Verification items for this drawing (mm, ordinates from the low corner). A direction names the side the tool comes from. Round coordinates to 2 decimals unless told otherwise and drop trailing zeros. Loops run counter-clockwise (first coordinate to the right, second up) from the corner with the lowest first, then second, coordinate; pieces in that order, holes last. Notation, with made-up numbers: M 42.25,37.5 L 93.25,37.5 A15 ccw 93.25,47.5 Z; hole C 54.5,41.25 d6. An arc over 180 degrees is marked long. One line per item, written item: value.
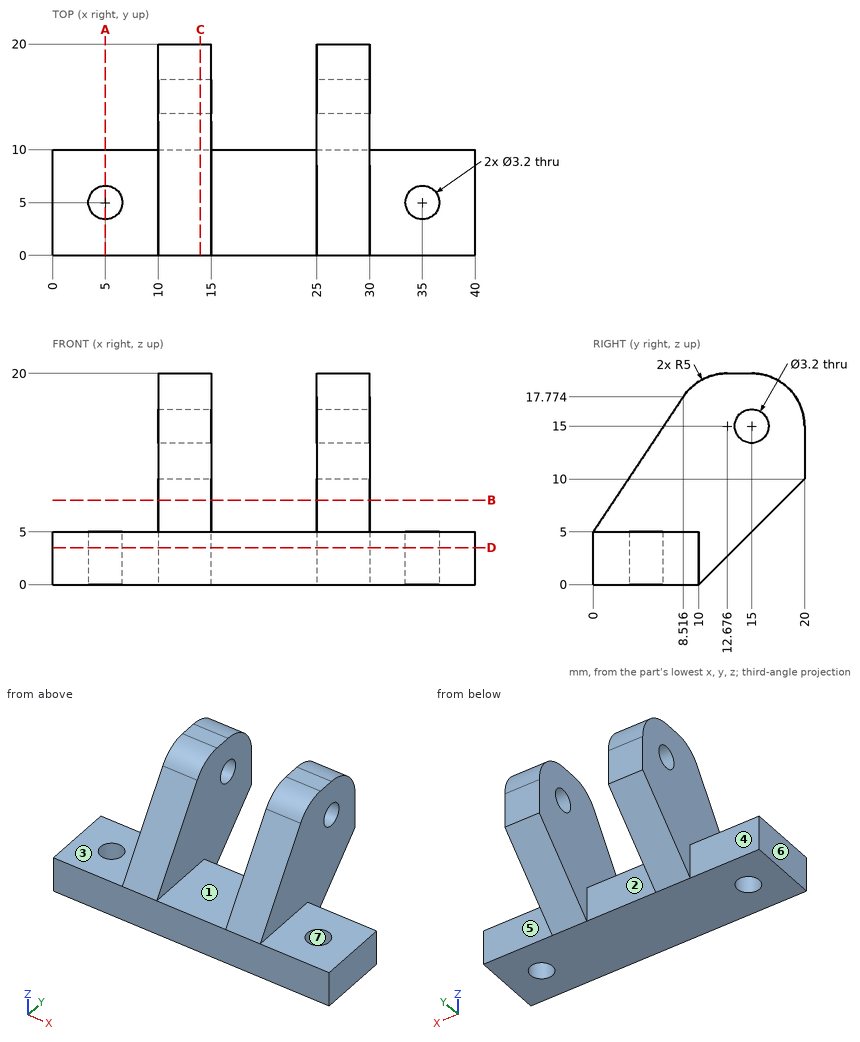
(1) Sectioned sample at C-C on x = 14. Enter the section's corners in (y, z) (1 decimal).
Completed:
outline: M 0,0 L 10,0 L 20,10 L 20,15 A5 ccw 15,20 L 12.7,20 A5 ccw 8.5,17.8 L 0,5 Z; hole C 15,15 d3.2
(2) Depth check by flat-ended pin: pin 1 Ø3 at (x, y) = (5.5, 3) entering from +Z; pin 2 Ø5.5 at (x, z) = (4, 1.5) entering from +Y; pin 3 Ø6 at (y, z) = (14, 9) entering from -X. Enter the tip coordinate at first touch or a pass-through.
Completed:
pin 1: stops at z = 5
pin 2: stops at y = 10
pin 3: stops at x = 10
(3) Sectioned sample at D-D on z = 3.5. Enter the section's corners in (x, y).
Completed:
outline: M 0,0 L 40,0 L 40,10 L 30,10 L 30,13.5 L 25,13.5 L 25,10 L 15,10 L 15,13.5 L 10,13.5 L 10,10 L 0,10 Z; hole C 5,5 d3.2; hole C 35,5 d3.2
(4) Thickness scan on L1, parallel to Y at x = 5, z = 1.5; L2, parallel to X at y = 4.5, z = 9; L3, parallel to Z at x = 8, y = 1.75. Record the ranges inside material, lowest first. Write a range as from..to.
Completed:
L1: y = 0..3.4, 6.6..10
L2: x = 10..15, 25..30
L3: z = 0..5
(5) Mould release check, pull along X, two halves, no side actions. Record for the marked faces 5, 6 and 7: +X half, -X half, draft (parallel to the pull), parting line (faces both ways), or undercut.
Completed:
face 5: draft
face 6: -X half
face 7: undercut
(6) Sectioned sample at A-A on x = 5. Enter the section's corners in (y, z), and give its area (3 significant figures).
Completed:
outline: M 0,0 L 3.4,0 L 3.4,5 L 0,5 Z; M 6.6,0 L 10,0 L 10,5 L 6.6,5 Z
area: 34.0 mm^2
(7) Tool access check on the marked faces 1, 2, 3 and 4. Record the directions out of +Z, -Z, +X, -X, +Y, -Y that give a thin tool (end or side, any length) a straight path to the whole face; none if there is none.
Completed:
face 1: +Z, +Y, -Y
face 2: +Z, -Z, +Y
face 3: +Z, -X, +Y, -Y
face 4: +Z, -Z, -X, +Y
(8) Sectioned sample at B-B on z = 8. Enter the section's corners in (x, y), and give its area (3 significant figures).
Completed:
outline: M 10,2 L 15,2 L 15,18 L 10,18 Z; M 25,2 L 30,2 L 30,18 L 25,18 Z
area: 160 mm^2
